```python
from build123d import *

# Parameters (mm, degrees)
F1_DEPTH = 5
F3_D     = 4
F4_D     = 4.1
F5_D     = 4.2
F6_D     = 4.3
F7_D     = 4.4
F8_D     = 3.9
F9_D     = 3.8
F10_D    = 3.7
F11_D    = 3.6


with BuildPart() as f1:
    # F0 (on Front) → F1 (new body)
    with BuildSketch(Plane.XZ):
        Polygon((100, -25), (100, 25), (-100, 25), (-100, -25), (-89.7911712527, -25), (-89.7911712527, -5), (-85.2911712527, -5), (-85.2911712527, -25), (-77.3481056094, -25), (-77.3481056094, -5), (-72.7481056094, -5), (-72.7481056094, -25), (-62.5451430678, -25), (-62.5451430678, -5), (-57.8451430678, -5), (-57.8451430678, -25), (-43.0224016309, -25), (-43.0224016309, -5), (-38.2224016309, -5), (-38.2224016309, -25), (-25.8595496416, -25), (-25.8595496416, -5), (-20.9595496416, -5), (-20.9595496416, -25), (-3.3333026804, -25), (-3.3333026804, -5), (1.6666973196, -5), (1.6666973196, -25), (10.6115136296, -25), (10.6115136296, -5), (15.7115136296, -5), (15.7115136296, -25), (26.4871511608, -25), (26.4871511608, -5), (31.6871511608, -5), (31.6871511608, -25), (44.50815171, -25), (44.50815171, -5), (49.80815171, -5), (49.80815171, -25), (57.3802888393, -25), (57.3802888393, -5), (62.7802888393, -5), (62.7802888393, -25), (72.8268548846, -25), (72.8268548846, -5), (78.3268548846, -5), (78.3268548846, -25), align=None)
    extrude(amount=F1_DEPTH)

    # F3 (through all)
    with Locations(Plane(origin=(0, 0, 0), x_dir=(1, 0, 0), z_dir=(0, 1, 0))):
        with Locations((0, -14.6358385682)):
            Hole(F3_D / 2)

    # F4 (through all)
    with Locations(Plane(origin=(0, 0, 0), x_dir=(1, 0, 0), z_dir=(0, 1, 0))):
        with Locations((20, -14.6358385682)):
            Hole(F4_D / 2)

    # F5 (through all)
    with Locations(Plane(origin=(0, 0, 0), x_dir=(1, 0, 0), z_dir=(0, 1, 0))):
        with Locations((40, -14.6358385682)):
            Hole(F5_D / 2)

    # F6 (through all)
    with Locations(Plane(origin=(0, 0, 0), x_dir=(1, 0, 0), z_dir=(0, 1, 0))):
        with Locations((60, -14.6358385682)):
            Hole(F6_D / 2)

    # F7 (through all)
    with Locations(Plane(origin=(0, 0, 0), x_dir=(1, 0, 0), z_dir=(0, 1, 0))):
        with Locations((80, -14.6358385682)):
            Hole(F7_D / 2)

    # F8 (through all)
    with Locations(Plane(origin=(0, 0, 0), x_dir=(1, 0, 0), z_dir=(0, 1, 0))):
        with Locations((-20, -14.6358385682)):
            Hole(F8_D / 2)

    # F9 (through all)
    with Locations(Plane(origin=(0, 0, 0), x_dir=(1, 0, 0), z_dir=(0, 1, 0))):
        with Locations((-40, -14.6358385682)):
            Hole(F9_D / 2)

    # F10 (through all)
    with Locations(Plane(origin=(0, 0, 0), x_dir=(1, 0, 0), z_dir=(0, 1, 0))):
        with Locations((-60, -14.6358385682)):
            Hole(F10_D / 2)

    # F11 (through all)
    with Locations(Plane(origin=(0, 0, 0), x_dir=(1, 0, 0), z_dir=(0, 1, 0))):
        with Locations((-80, -14.6358385682)):
            Hole(F11_D / 2)


solid = f1.part
```
The model under review builds one solid part; all positions refer to its coordinate system, in mm. A direction names the side the tool comes from. Round coordinates to 2 decimals unless told otherwise and drop trailing zeros. Loops run counter-clockwise (first coordinate to the right, second up) from the corner with the lowest first, then second, coordinate; pieces in that order, holes last. Notation, with made-up numbers: (-20, 87) - (-13, 87) arc R34 cw to (-13, 120) - close; hole circle Ø4 at (-4, 29). An arc over 180 degrees is marked (long way). Use a Markdown table: item, result. Add a question column.
Q1. Add section B-B (x = 20). State the section outline as (y, z) points.
Q2. Insertion check: pin 1 Ø2 at (x, z) = (-80, 14.64) entering from +Y. The pin has a flat end and moves straight along its axis. Give the tip position at first contact, or say it passes through.
Q3. Add section C-C (z = -13). State how many separate pieces and enclosed holes the cut face has, plus the area to 3 significant figures.
Q4. The part is to be moulded in two halves that separate along X. For faces 3 (the face through (1, -2, 25)), 4 (the face through (-85.291, -2, -15)), say which applies: pulls with the +X half, pulls with the -X half, needs draft (parallel to the pull), parting line crosses it, or undercut.
Q5. For probe 1 along Z at (x, y) = (80, -2.8); probe 2 along Z at (x, y) = (20, -3.25), list the stretches that pass through material, from the lowest coordinate up.
Q6. Add section A-A (x = -60). State the section outline as (y, z) points.
Q7. Machinability: for faces 1 (the face through (-95, -2, -25)), 2 (the face through (78.327, -2, -15)), which of the approach directions +Z, -Z, +X, -X, +Y, -Y give a long, thin tool a straight path to every point of the face, cutting with its end or side? Answer none if there is none.
Worked answers:
| question | item | result |
|---|---|---|
| 1 | outline | (-5, -25) - (0, -25) - (0, 12.59) - (-5, 12.59) - close; (-5, 16.69) - (0, 16.69) - (0, 25) - (-5, 25) - close |
| 2 | pin 1 | through |
| 3 | separate pieces | 12 |
| 3 | enclosed holes | 0 |
| 3 | area | 725 mm² |
| 4 | face 3 | needs draft |
| 4 | face 4 | undercut |
| 5 | probe 1 | -25 to 12.44, 16.84 to 25 |
| 5 | probe 2 | -25 to 12.59, 16.69 to 25 |
| 6 | outline | (-5, -5) - (0, -5) - (0, 12.79) - (-5, 12.79) - close; (-5, 16.49) - (0, 16.49) - (0, 25) - (-5, 25) - close |
| 7 | face 1 | -Z, +X, -X, +Y, -Y |
| 7 | face 2 | -Z, +Y, -Y |
